```python
from build123d import *
from OCP.BRepFilletAPI import BRepFilletAPI_MakeChamfer

# Parameters (mm, degrees)
SKETCH1_R           = 15
BOSS_EXTRUDE1_DEPTH = 176.241933
SKETCH2_R           = 7.383069666
CUT_EXTRUDE1_DEPTH  = 178.513996484
CHAMFER1_SIZE       = 1.330296
CHAMFER1_SIZE2      = 1.0719


with BuildPart() as part:
    # Sketch1 → Boss-Extrude1 (new body)
    with BuildSketch(Plane(origin=(0, 0, 0), x_dir=(1, 0, 0), z_dir=(0, 1, 0))):
        with Locations(Location((0, 0, 0), (0, 0, 270))):
            Circle(SKETCH1_R)
    extrude(amount=BOSS_EXTRUDE1_DEPTH)

    # Sketch2 → Cut-Extrude1 (cut, through all)
    with BuildSketch(Plane(origin=(0, 0, 0), x_dir=(1, 0, 0), z_dir=(0, 1, 0))):
        with Locations(Location((0, 0, 0), (0, 0, 270))):
            Circle(SKETCH2_R)
    extrude(amount=CUT_EXTRUDE1_DEPTH, mode=Mode.SUBTRACT)

    # Chamfer1: one chamfer whose edges measure the first distance from different faces: ONE call of the kernel's chamfer builder (chamfer() names one face for all edges)
    chamfer1_edges_1 = [part.edges().sort_by_distance(p)[0] for p in [
        (0, 0, -15),
    ]]
    chamfer1_side_1 = [part.faces().sort_by_distance(p)[0] for p in [
        (0, 0, -14.575735931),
    ]]
    chamfer1_edges_2 = [part.edges().sort_by_distance(p)[0] for p in [
        (0, 176.241933, -15),
    ]]
    chamfer1_side_2 = [part.faces().sort_by_distance(p)[0] for p in [
        (0, 88.1209665, -15),
    ]]
    chamfer1 = BRepFilletAPI_MakeChamfer(part.part.solid().wrapped)
    for e in chamfer1_edges_1:
        chamfer1.Add(CHAMFER1_SIZE, CHAMFER1_SIZE2, e.wrapped, chamfer1_side_1[0].wrapped)  # the first distance lies on this face
    for e in chamfer1_edges_2:
        chamfer1.Add(CHAMFER1_SIZE, CHAMFER1_SIZE2, e.wrapped, chamfer1_side_2[0].wrapped)  # the first distance lies on this face
    add(Compound.cast(chamfer1.Shape()), mode=Mode.REPLACE)


solid = part.part
```
Input: part model. Units: mm. Frame: model coordinates. Coordinates: 2 decimals unless noted, no trailing zeros. Write each loop counter-clockwise with the first axis right and the second up, starting at its lowest first coordinate (ties: lowest second). Pieces come first, ordered by that corner, then holes.
1) Section C-C on y = 112. Output: boundary loops of the cut face in (x, z), and give its area (3 significant figures).
2) Material intervals for line 1 along X through (y, z) = (122.5, 0); line 2 along Z through (x, y) = (-4, 149.5); line 3 along X through (y, z) = (106.5, 5), sorted ascending.
3) Section B-B on z = 0. Output: boundary loops of the cut face in (x, y), and give its area (3 significant figures).
4) Mould query, pull axis X, two halves, no side actions, for faces 1 (the flat face through (-6, 176.242, 6)), 2 (the cylindrical face through (0.66, 86.775, -14.985)), 3 (the cylindrical face through (0.325, 86.887, -7.376)). Classes: pulls with the +X half, pulls with the -X half, needs draft (parallel to the pull), parting line crosses it, or undercut.
5) Section A-A on x = 0. Output: boundary loops of the cut face in (y, z), and give its area (3 significant figures).
6) Pin query (flat end, axial travel): pin 1 Ø8 at (x, y) = (-4, 97) entering from +Z; pin 2 Ø10 at (x, y) = (-10.5, 121) entering from +Z; pin 3 Ø1 at (x, y) = (5, 37) entering from -Z; pin 4 Ø3 at (y, z) = (104.5, -9.5) entering from +X. Return the tip coordinate at first contact, or that it passes through.
Check result:
1. outline: circle Ø30 at (0, 0); hole circle Ø14.77 at (0, 0)
1. area: 536 mm2
2. line 1: x = -15 to -7.38, 7.38 to 15
2. line 2: z = -14.46 to -6.21, 6.21 to 14.46
2. line 3: x = -14.14 to -5.43, 5.43 to 14.14
3. outline: (-15, 1.07) - (-13.67, 0) - (-7.38, 0) - (-7.38, 176.24) - (-13.93, 176.24) - (-15, 174.91) - close; (7.38, 0) - (13.67, 0) - (15, 1.07) - (15, 174.91) - (13.93, 176.24) - (7.38, 176.24) - close
3. area: 2,680 mm2
4. face 1: needs draft
4. face 2: parting line crosses it
4. face 3: undercut
5. outline: (0, -13.67) - (1.07, -15) - (174.91, -15) - (176.24, -13.93) - (176.24, -7.38) - (0, -7.38) - close; (0, 7.38) - (176.24, 7.38) - (176.24, 13.93) - (174.91, 15) - (1.07, 15) - (0, 13.67) - close
5. area: 2,680 mm2
6. pin 1: stops at z = 15
6. pin 2: stops at z = 13.96
6. pin 3: stops at z = -14.31
6. pin 4: stops at x = 12.69
